```python
from build123d import *

# Parameters (mm, degrees)
EXTRUDE_1_DEPTH = 480
SCALE_1_SCALE   = 1.3


with BuildPart() as part:
    # 草图1 → 凸台-拉伸1 (new body)
    with BuildSketch(Plane.XY):
        with BuildLine():
            Line((-7619.991111067, 5536), (-7139.991111067, 5536))
            ThreePointArc((-7139.991111067, 5536), (-6989.477063432, 5607.677609574), (-6833.3126292, 5666.028511287))
            Line((-6833.3126292, 5666.028511287), (-6928.829756014, 5960))
            Line((-6928.829756014, 5960), (-7619.991111067, 5960))
            Line((-7619.991111067, 5960), (-7619.991111067, 5536))
        make_face()
    extrude(amount=EXTRUDE_1_DEPTH)


with BuildPart() as part_1:
    # 缩放比例1: scaled about (0, 0, 0)
    add(part.part.scale(SCALE_1_SCALE))


solid = part_1.part
```
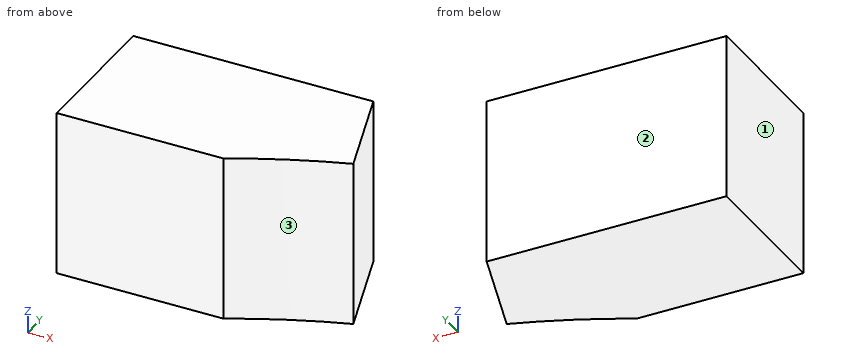
The model under review builds one solid part; all positions refer to its coordinate system, in mm. Face numbers are marked on the shaded views. Coordinates: 2 decimals unless noted, no trailing zeros. Write each loop counter-clockwise with the first axis right and the second up, starting at its lowest first coordinate (ties: lowest second). Pieces come first, ordered by that corner, then holes.
1) We need section C-C on x = -9181.5. State the section outline as (y, z) points, then the cut area to 3 significant figures.
2) To check wall thickness, follow probe 1 along Y at (x, z) = (-9265, 69.5); probe 2 along X at (y, z) = (7519, 576); probe 3 along X at (y, z) = (7540, 332). State the ranges of each line that lie inside material, in increasing order.
3) Clearance check with flat-ended pins moving along their axes: pin 1 Ø1.5 at (y, z) = (7480, 178) entering from +X; pin 2 Ø5 at (y, z) = (7555, 180.5) entering from +X; pin 3 Ø3 at (y, z) = (7661.5, 295) entering from +X. State where each tip first meets the part, or that it passes through.
4) We need section B-B on y = 7608.5. State the section outline as (x, z) points.
5) The part is to be moulded in two halves that separate along Y. For the marked faces 1, 2 and 3, say which applies: pulls with the +Y half, pulls with the -Y half, needs draft (parallel to the pull), parting line crosses it, or undercut.
6) We need section A-A on z = 455. State the section outline as (x, y) points, then the cut area to 3 significant figures.
Answer list:
1. outline: (7247.26, 0) - (7748, 0) - (7748, 624) - (7247.26, 624) - close
1. area: 312,000 mm2
2. probe 1: y = 7205.73 to 7748
2. probe 2: x = -9905.99 to -8933.07
2. probe 3: x = -9905.99 to -8939.9
3. pin 1: stops at x = -8920.16
3. pin 2: stops at x = -8943.96
3. pin 3: stops at x = -8978.89
4. outline: (-9905.99, 0) - (-8962.15, 0) - (-8962.15, 624) - (-9905.99, 624) - close
5. face 1: needs draft
5. face 2: pulls with the +Y half
5. face 3: pulls with the -Y half
6. outline: (-9905.99, 7196.8) - (-9281.99, 7196.8) arc R2496 cw to (-8883.31, 7365.84) - (-9007.48, 7748) - (-9905.99, 7748) - close
6. area: 504,000 mm2
